```python
from build123d import *

# Parameters (mm, degrees)
CROQUIS2_W              = 30.3
CROQUIS2_H              = 70
SALIENTE_EXTRUIR2_DEPTH = 5
SALIENTE_EXTRUIR3_START = -20
SALIENTE_EXTRUIR3_DEPTH = 70
SALIENTE_EXTRUIR4_START = -20
CROQUIS4_W              = 20.2
CROQUIS4_H              = 20.2
SALIENTE_EXTRUIR4_DEPTH = 4
CHAFL_N4_SIZE           = 4
CROQUIS6_W              = 30.3
CROQUIS6_H              = 5
CROQUIS6_W_2            = 5.125
CROQUIS6_H_2            = 40.5
SALIENTE_EXTRUIR6_DEPTH = 40
SALIENTE_EXTRUIR7_START = -15.15
SALIENTE_EXTRUIR7_DEPTH = 30.3
CROQUIS8_W              = 22.3
CROQUIS8_H              = 24.5
CORTAR_EXTRUIR1_DEPTH   = 40
CHAFL_N7_SIZE           = 3
CHAFL_N7_SIZE2          = 11.196152423
CHAFL_N9_SIZE           = 5


with BuildPart() as part:
    # Croquis2 → Saliente-Extruir2 (new body)
    with BuildSketch(Plane.XY):
        with Locations((0, 15)):
            Rectangle(CROQUIS2_W, CROQUIS2_H)
    extrude(amount=-SALIENTE_EXTRUIR2_DEPTH)

    # Croquis3 → Saliente-Extruir3 (add)
    with BuildSketch(Plane(origin=(0, 0, 0), x_dir=(1, 0, 0), z_dir=(0, 1, 0)).offset(SALIENTE_EXTRUIR3_START)):
        Polygon((-15.15, 30.25), (-15.15, 5), (-10.1, 5), (-10.1, 25.2), (10.1, 25.2), (10.1, 5), (15.15, 5), (15.15, 30.25), align=None)
    extrude(amount=SALIENTE_EXTRUIR3_DEPTH)

    # Croquis4 → Saliente-Extruir4 (add)
    with BuildSketch(Plane(origin=(0, 0, 0), x_dir=(1, 0, 0), z_dir=(0, 1, 0)).offset(SALIENTE_EXTRUIR4_START)):
        with Locations((0, 15.1)):
            Rectangle(CROQUIS4_W, CROQUIS4_H)
    extrude(amount=SALIENTE_EXTRUIR4_DEPTH)

    # Chaflán4
    chafl_n4_edges = [part.edges().sort_by_distance(p)[0] for p in [
        (0, 50, -5),
        (10.1, 50, -15.1),
        (0, 50, -25.2),
        (-10.1, 50, -15.1),
    ]]
    chamfer(chafl_n4_edges, length=CHAFL_N4_SIZE)

    # Croquis6 → Saliente-Extruir6 (add)
    with BuildSketch(Plane.XY):
        with Locations((0, 23)):
            Rectangle(CROQUIS6_W, CROQUIS6_H)
        with Locations((-12.5875, 0.25)):
            Rectangle(CROQUIS6_W_2, CROQUIS6_H_2)
        with Locations((12.5875, 0.25)):
            Rectangle(CROQUIS6_W_2, CROQUIS6_H_2)
    extrude(amount=SALIENTE_EXTRUIR6_DEPTH)

    # Croquis7 → Saliente-Extruir7 (add)
    with BuildSketch(Plane(origin=(0, 0, 0), x_dir=(0, 0, -1), z_dir=(1, 0, 0)).offset(SALIENTE_EXTRUIR7_START)):
        Polygon((-40, 25.5), (0, 50), (0, 25.5), align=None)
    extrude(amount=SALIENTE_EXTRUIR7_DEPTH)

    # Croquis8 → Cortar-Extruir1 (cut)
    with BuildSketch(Plane.XY):
        with Locations((0, 37.75)):
            Rectangle(CROQUIS8_W, CROQUIS8_H)
    extrude(amount=CORTAR_EXTRUIR1_DEPTH, mode=Mode.SUBTRACT)

    # Chaflán7
    chafl_n7_edges = [part.edges().sort_by_distance(p)[0] for p in [
        (-10.025, 0.25, 40),
        (0, 20.5, 40),
        (10.025, 0.25, 40),
    ]]
    chafl_n7_side = [part.faces().sort_by_distance(p)[0] for p in [
        (14.603342886, 2.75, 40),
    ]]
    chamfer(chafl_n7_edges, length=CHAFL_N7_SIZE, length2=CHAFL_N7_SIZE2, reference=chafl_n7_side[0])

    # Chaflán9
    chafl_n9_edges = [part.edges().sort_by_distance(p)[0] for p in [
        (10.025, -20, 14.401923789),
        (-10.025, -20, 14.401923789),
    ]]
    chamfer(chafl_n9_edges, length=CHAFL_N9_SIZE)


solid = part.part
```
Source: CAD feature listing. Evaluate the final solid. Frame: model axes, mm. A direction names the side the tool comes from. Give positions to 0.01 mm unless a question says otherwise; leave off trailing zeros. Loops run counter-clockwise (first coordinate to the right, second up) from the corner with the lowest first, then second, coordinate; pieces in that order, holes last. Notation, with made-up numbers: (-13.75, 7) -> (8.25, 7) arc R10 cw to (8.25, 11) -> close; hole circle Ø6 at (41.25, 77.25). An arc over 180 degrees is marked (long way). Put each result on its own line as item: value. Start each with the question number.
1) Cut plane A-A (z = 24). Return loops of the section in (x, y) (3 decimals).
2) Draft query along X for faces 1 (the face through (12.1, 48, -15.3)), 2 (the face through (13.12, 37.58, 20.28)), 3 (the face through (-0.2, 48, -27.2)), 4 (the face through (15.15, 15, 4)). Return one class per face: released by +X, released by -X, zero draft, split by the parting line, or undercut.
3) Contact query for flat-ended pins moving along their axis: P1, Ø16, axis at x = -4.5, z = 16, coming from the -Y side (3 decimals); P2, Ø10, axis at x = -0.5, z = -16, coming from the +Y side; P3, Ø3, axis at x = 7.5, z = 27.5, coming from the -Y side. Output: stop coordinate, or through.
4) Reachability of faces 5 (the face through (-12.49, -17.465, 19.72)), 6 (the face through (11.15, 35, 15)), 7 (the face through (0, 48, -3)), 8 (the face through (0, 15, -30.25)) from +Z, -Z, +X, -X, +Y, -Y: full face, straight path, thin tool, end or side. Return the list, or none.
5) Material intervals for probe 1 along X at (y, z) = (9, 17) (3 decimals); probe 2 along X at (y, z) = (42.5, -19.5); probe 3 along Z at (x, y) = (3, 11), sorted ascending.
6) Cut plane B-B (y = 6.5). Return loops of the section in (x, z) (3 decimals).
7) Cut plane D-D (y = 44.5). Return loops of the section in (x, z), then the cut area to 3 significant figures.
8) Cut plane C-C (x = -4). Return loops of the section in (y, z), then the cut area to 3 significant figures.
Results are:
1. outline: (-15.15, -20) -> (-15.025, -20) -> (-10.025, -15) -> (-10.025, 20.5) -> (10.025, 20.5) -> (10.025, -15) -> (15.025, -20) -> (15.15, -20) -> (15.15, 35.3) -> (11.15, 35.3) -> (11.15, 25.5) -> (-11.15, 25.5) -> (-11.15, 35.3) -> (-15.15, 35.3) -> close
2. face 1: undercut
2. face 2: zero draft
2. face 3: undercut
2. face 4: released by +X
3. P1: stops at y = -17.475
3. P2: stops at y = -16
3. P3: stops at y = 20.5
4. face 5: +Z, -Y
4. face 6: +Z, +Y
4. face 7: +Y
4. face 8: -Z, +X, -X, +Y, -Y
5. probe 1: x = -15.15 to -10.025, 10.025 to 15.15
5. probe 2: x = -15.15 to -10.1, 10.1 to 15.15
5. probe 3: z = -30.25 to -25.2, -5 to 0
6. outline: (-15.15, -30.25) -> (15.15, -30.25) -> (15.15, 40) -> (13.025, 40) -> (10.025, 28.804) -> (10.025, 0) -> (-10.025, 0) -> (-10.025, 28.804) -> (-13.025, 40) -> (-15.15, 40) -> close; hole (-10.1, -25.2) -> (10.1, -25.2) -> (10.1, -5) -> (-10.1, -5) -> close
7. outline: (-15.15, -30.25) -> (15.15, -30.25) -> (15.15, 8.98) -> (11.15, 8.98) -> (11.15, 0) -> (-11.15, 0) -> (-11.15, 8.98) -> (-15.15, 8.98) -> close; hole (-10.1, -25.2) -> (10.1, -25.2) -> (10.1, -5) -> (-10.1, -5) -> close
7. area: 580 mm2
8. outline: (-20, -30.25) -> (50, -30.25) -> (50, -29.2) -> (46, -25.2) -> (-16, -25.2) -> (-16, -5) -> (46, -5) -> (50, -1) -> (50, 0) -> (25.5, 0) -> (25.5, 40) -> (23.5, 40) -> (20.5, 28.8) -> (20.5, 0) -> (-20, 0) -> close
8. area: 952 mm2
